from build123d import *

# Parameters (mm, degrees)
F0_R     = 50.8
F1_DEPTH = 25.4
F2_R     = 10.16
F3_DEPTH = 12.7
F4_DEPTH = 12.7
F5_R     = 12.7
F6_DEPTH = 44.45


with BuildPart() as f1:
    # F0 (on Front) → F1 (new body, symmetric)
    with BuildSketch(Plane.XZ):
        Circle(F0_R)
    extrude(amount=F1_DEPTH, both=True)

    # F2
    f2_edges = [f1.edges().sort_by_distance(p)[0] for p in [
        (-50.8, -25.4, 0),
        (-50.8, 25.4, 0),
    ]]
    fillet(f2_edges, radius=F2_R)

    # F3 (cut): faces of the model
    f3_faces = [f1.faces().sort_by_distance(p)[0] for p in [
        (0, -25.4, 0),
        (0, 25.4, 0),
    ]]
    extrude(f3_faces, amount=F3_DEPTH, dir=(0, -1, 0), mode=Mode.SUBTRACT)

    # F4 (cut): a face of the model
    f4_faces = [f1.faces().sort_by_distance(p)[0] for p in [
        (0, -25.4, 0),
    ]]
    extrude(f4_faces, amount=-F4_DEPTH, mode=Mode.SUBTRACT)

    # F5 (on Front) → F6 (join, symmetric)
    with BuildSketch(Plane.XZ):
        Circle(F5_R)
    extrude(amount=F6_DEPTH, both=True)


solid = f1.part
Check sheet for the modelled part. Datum: model origin and axes. Units: mm. A direction names the side the tool comes from. Coordinates: 2 decimals unless noted, no trailing zeros. Write each loop counter-clockwise with the first axis right and the second up, starting at its lowest first coordinate (ties: lowest second). Pieces come first, ordered by that corner, then holes.
Item 1: Cross-section at C-C on y = -22. Record the boundary of the cut face in (x, z), then the cut area to 3 significant figures.
Numbers:
outline: circle Ø96.45 at (0, 0); circle Ø25.4 at (0, 0); hole circle Ø81.28 at (0, 0)
area: 2,620 mm2
Item 2: Scan lines: probe 1 along Z at (x, y) = (0, -15.5); probe 2 along Z at (x, y) = (0, 18); probe 3 along Y at (x, z) = (-8.5, -21). Record each from-to range of solid material in increasing order.
Numbers:
probe 1: z = -50.8 to -40.64, -12.7 to 12.7, 40.64 to 50.8
probe 2: z = -50.42 to -40.64, -12.7 to 12.7, 40.64 to 50.42
probe 3: y = -12.7 to 12.7
Item 3: Access from +Z, -Z, +X, -X, +Y, -Y to the whole of each face (thin tool, end or side, straight path). Record for faces 5 (the face through (-10, -12.7, 10)), 6 (the face through (0, -44.45, 0)), 7 (the face through (-10, 12.7, 10)).
Numbers:
face 5: -Y
face 6: +Z, -Z, +X, -X, -Y
face 7: +Y
Item 4: Cross-section at D-D on y = -2.5. Record the boundary of the cut face in (x, z).
Numbers:
outline: circle Ø101.6 at (0, 0)
Item 5: Cross-section at A-A on x = 0. Record the boundary of the cut face in (y, z), then the cut area to 3 significant figures.
Numbers:
outline: (-44.45, -12.7) - (-12.7, -12.7) - (-12.7, -40.64) - (-25.4, -40.64) arc R10.16 ccw to (-15.24, -50.8) - (15.24, -50.8) arc R10.16 ccw to (25.4, -40.64) - (12.7, -40.64) - (12.7, -12.7) - (44.45, -12.7) - (44.45, 12.7) - (12.7, 12.7) - (12.7, 40.64) - (25.4, 40.64) arc R10.16 ccw to (15.24, 50.8) - (-15.24, 50.8) arc R10.16 ccw to (-25.4, 40.64) - (-12.7, 40.64) - (-12.7, 12.7) - (-44.45, 12.7) - close
area: 4,620 mm2
Item 6: Mould release check, pull along X, two halves, no side actions. Record for faces 1 (the face through (0, 44.45, 0)), 2 (the face through (-11.012, -0.213, -49.592)), 3 (the face through (-2.75, 28.35, -12.4)), 4 (the face through (-5.291, 19.139, 40.294)): released by +X, released by -X, zero draft, split by the parting line, or undercut.
Numbers:
face 1: zero draft
face 2: split by the parting line
face 3: undercut
face 4: undercut
Item 7: Cross-section at B-B on z = 0. Record the boundary of the cut face in (x, y), then the cut area to 3 significant figures.
Numbers:
outline: (-50.8, -15.24) arc R10.16 ccw to (-40.64, -25.4) - (-40.64, -12.7) - (-12.7, -12.7) - (-12.7, -44.45) - (12.7, -44.45) - (12.7, -12.7) - (40.64, -12.7) - (40.64, -25.4) arc R10.16 ccw to (50.8, -15.24) - (50.8, 15.24) arc R10.16 ccw to (40.64, 25.4) - (40.64, 12.7) - (12.7, 12.7) - (12.7, 44.45) - (-12.7, 44.45) - (-12.7, 12.7) - (-40.64, 12.7) - (-40.64, 25.4) arc R10.16 ccw to (-50.8, 15.24) - close
area: 4,620 mm2
Item 8: Depth check by flat-ended pin: pin 1 Ø8 at (x, z) = (-21, 26.5) entering from +Y; pin 2 Ø8 at (x, y) = (-25.5, -17) entering from -Z; pin 3 Ø8 at (y, z) = (-29.5, -11.5) entering from -X. Enter the tip coordinate at first touch or a pass-through.
Numbers:
pin 1: stops at y = 12.7
pin 2: stops at z = -45.94
pin 3: stops at x = -10.25
